```python
from build123d import *

# Parameters (mm, degrees)
BOSS_EXTRUDE1_DEPTH = 1.524


with BuildPart() as part:
    # Sketch1 → Boss-Extrude1 (new body)
    with BuildSketch(Plane.XY):
        with BuildLine():
            Line((25.018211481, 1.458274504), (28.403024501, 2.465831103))
            Line((28.403024501, 2.465831103), (28.147078807, 3.040199114))
            ThreePointArc((28.147078807, 3.040199114), (31.031837949, 3.343352077), (33.541663921, 1.889216381))
            Line((33.541663921, 1.889216381), (32.890976581, 1.164259908))
            Line((32.890976581, 1.164259908), (34.272042889, -0.07532122))
            Line((34.272042889, -0.07532122), (32.226452866, 0.530981017))
            ThreePointArc((32.226452866, 0.530981017), (30.745835594, 1.027103578), (29.265218322, 0.530981017))
            Line((29.265218322, 0.530981017), (29.028606423, 1.061962035))
            Line((29.028606423, 1.061962035), (25.453006053, -0.002386196))
            ThreePointArc((25.453006053, -0.002386196), (23.593059825, 0.239006946), (25.018211481, 1.458274504))
        make_face()
    extrude(amount=-BOSS_EXTRUDE1_DEPTH)


solid = part.part
```
The model under review builds one solid part; all positions refer to its coordinate system, in mm. A direction names the side the tool comes from. Round coordinates to 2 decimals unless told otherwise and drop trailing zeros. Order: outer loops, then holes, each group sorted by start corner. A loop starts at its lowest first (then second) coordinate and runs counter-clockwise, first axis right, second up. Notation, with made-up numbers: (33, -38) -> (39, -38) arc R20 ccw to (39, -17) -> close; hole circle Ø11 at (87.5, 23.25). An arc over 180 degrees is marked (long way). Use a Markdown table: item, result.
Q1. Tool access review of faces 1 (the flat face through (33.572, 0.553, -0.751)), 2 (the flat face through (29, 2, 0)), 3 (the flat face through (33.264, 0.224, -0.751)): name each direction out of +Z, -Z, +X, -X, +Y, -Y from which nothing blocks a thin tool from reaching the whole face with its end or side.
Values:
| item | result |
|---|---|
| face 1 | +Z, -Z, +X |
| face 2 | +Z, +X, -X, +Y, -Y |
| face 3 | +Z, -Z, -Y |
Q2. For line 1 (Y direction, x = 28.25, z = -0.9); line 2 (Y direction, x = 33, z = -1.35); line 3 (Y direction, x = 31, z = -1.1), list the stretches that pass through material, from the lowest coordinate up.
Values:
| item | result |
|---|---|
| line 1 | y = 0.83 to 2.42, 2.81 to 3.08 |
| line 2 | y = 0.3 to 1.07, 1.29 to 2.4 |
| line 3 | y = 1.01 to 3.35 |
Q3. We need section B-B on y = 0.25. Write out the cut boundary in (x, z), then the cut area to 3 significant figures.
Values:
| item | result |
|---|---|
| outline | (23.59, -1.52) -> (26.3, -1.52) -> (26.3, 0) -> (23.59, 0) -> close; (33.17, -1.52) -> (33.91, -1.52) -> (33.91, 0) -> (33.17, 0) -> close |
| area | 5.25 mm^2 |
Q4. Clearance check with a flat-ended pin moving along its axis: P1, Ø2, axis at x = 29, y = 0, coming from the -Z side. State where the tip first meets the part, or that it passes through.
Values:
| item | result |
|---|---|
| P1 | stops at z = -1.52 |
Q5. Mouldability with a two-part tool opening along X and no side actions: class faces 4 (the flat face through (29, 2, -1.524)), 5 (the cylindrical face through (30.991, 3.352, -0.751)), 6 (the flat face through (27.27, 0.54, -0.75)) as +X half, -X half, draft (parallel to the pull), parting line (faces both ways), or undercut.
Values:
| item | result |
|---|---|
| face 4 | draft |
| face 5 | parting line |
| face 6 | undercut |
Q6. We need section D-D on x = 29.75. Write out the cut boundary in (y, z).
Values:
| item | result |
|---|---|
| outline | (0.82, -1.52) -> (3.44, -1.52) -> (3.44, 0) -> (0.82, 0) -> close |
Q7. We need section A-A on z = -0.3. Write out the cut boundary in (x, y).
Values:
| item | result |
|---|---|
| outline | (25.02, 1.46) arc R1.03 ccw (long way) to (25.45, 0) -> (29.03, 1.06) -> (29.27, 0.53) arc R2.46 cw to (32.23, 0.53) -> (34.27, -0.08) -> (32.89, 1.16) -> (33.54, 1.89) arc R4.68 ccw to (28.15, 3.04) -> (28.4, 2.47) -> close |
Q8. We need section C-C on y = 0.7. Write out the cut boundary in (x, z).
Values:
| item | result |
|---|---|
| outline | (23.56, -1.52) -> (27.81, -1.52) -> (27.81, 0) -> (23.56, 0) -> close; (29.19, -1.52) -> (29.52, -1.52) -> (29.52, 0) -> (29.19, 0) -> close; (31.97, -1.52) -> (33.41, -1.52) -> (33.41, 0) -> (31.97, 0) -> close |
